Read the model definition and answer for the solid it produces. Units are mm, in the model's axes. Give positions to 0.01 mm unless a question says otherwise; leave off trailing zeros. Loops run counter-clockwise (first coordinate to the right, second up) from the corner with the lowest first, then second, coordinate; pieces in that order, holes last. Notation, with made-up numbers: (-25.5, -13) - (-15.5, -13) arc R18 ccw to (-15.5, 11) - close; hole circle Ø7 at (35, -37.75). An arc over 180 degrees is marked (long way). Put each result on its own line as item: value. Start each with the question number.
1. A cutting plane is placed at A-A, the plane y = 27. Determine the outline of the cut face in (x, z), plus the area to 3 significant figures.
2. Consider L1, parallel to Y at x = 0.45, z = -5.5; L2, parallel to Z at x = 0.5, y = 58.5; L3, parallel to Y at x = 0.95, z = -70.5. Determine where each line is inside the solid, lowest interval first. Write a range as from..to.
3. For a pull along Y with two mould halves and no side action, classify faces 1 (the flat face through (1.5, 15.6, -45.2)), 2 (the flat face through (0.76, 51.077, -11.662)) as released by +Y, released by -Y, zero draft, split by the parting line, or undercut.
4. A cutting plane is placed at C-C, the plane y = 63. Determine the outline of the cut face in (x, z), plus the area to 3 significant figures.
5. A cutting plane is placed at B-B, the plane x = 1.1. Count the separate pieces of the cut face and the enclosed holes in it, plus the area to 3 significant figures.
6. Given pin 1 Ø0.8 at (x, z) = (0.5, -44.5) entering from +Y, flat-ended and moving along its own axis, determine where the tip first touches the part or whether it passes through.
```python
from build123d import *

# Parameters (mm, degrees)
SKETCH1_R           = 1.05
BOSS_EXTRUDE1_DEPTH = 1.5
FILLET1_R           = 1.5
SKETCH2_W           = 117
SKETCH2_H           = 16
BOSS_EXTRUDE2_DEPTH = 1.5
CUT_EXTRUDE2_DEPTH  = 140.253366207
FILLET3_R           = 1
CUT_EXTRUDE3_DEPTH  = 140.253366207
BOSS_EXTRUDE3_DEPTH = 1.5
FILLET5_R           = 1.5


with BuildPart() as part:
    # Sketch1 → Boss-Extrude1 (new body)
    with BuildSketch(Plane(origin=(0, 0, 0), x_dir=(0, 0, -1), z_dir=(1, 0, 0))):
        Polygon((0, 0), (0, 75.5), (21.5, 75.5), (40, 0), (35.881667859, 0), (29.755840045, 25), (4, 25), (4, 0), align=None)
        with Locations((5.5, 72.5)):
            Circle(SKETCH1_R, mode=Mode.SUBTRACT)
        with Locations((18.5, 72.5)):
            Circle(SKETCH1_R, mode=Mode.SUBTRACT)
        Polygon((4, 69.5), (18.851866535, 69.5), (4, 29), align=None, mode=Mode.SUBTRACT)
        Polygon((8.260475549, 29), (20.558388216, 62.535546651), (28.775707595, 29), align=None, mode=Mode.SUBTRACT)
    extrude(amount=BOSS_EXTRUDE1_DEPTH)

    # Fillet1
    fillet1_edges = [part.edges().sort_by_distance(p)[0] for p in [
        (0.75, 75.5, -21.5),
        (0.75, 25, -29.755840045),
        (0.75, 25, -4),
        (0.75, 69.5, -4),
        (0.75, 29, -4),
        (0.75, 69.5, -18.851866535),
        (0.75, 29, -8.260475549),
        (0.75, 29, -28.775707595),
        (0.75, 62.535546651, -20.558388216),
    ]]
    fillet(fillet1_edges, radius=FILLET1_R)

    # Sketch2 → Boss-Extrude2 (add)
    with BuildSketch(Plane(origin=(1.5, 0, 0), x_dir=(0, 0, -1), z_dir=(1, 0, 0))):
        with Locations((58.5, 8)):
            Rectangle(SKETCH2_W, SKETCH2_H)
    extrude(amount=-BOSS_EXTRUDE2_DEPTH)

    # Sketch5 → Cut-Extrude2 (cut, through all)
    with BuildSketch(Plane(origin=(1.5, 0, 0), x_dir=(0, 0, -1), z_dir=(1, 0, 0))):
        Polygon((4.5, 11.5), (15.827584811, 11.5), (4.5, 5.626437506), align=None)
        Polygon((112.5, 11.5), (112.5, 5.626437506), (101.172415189, 11.5), align=None)
        Polygon((6.672415189, 4.5), (29.327584811, 4.5), (18, 10.373562494), align=None)
        Polygon((33.672415189, 4.5), (56.327584811, 4.5), (45, 10.373562494), align=None)
        Polygon((60.672415189, 4.5), (83.327584811, 4.5), (72, 10.373562494), align=None)
        Polygon((87.672415189, 4.5), (110.327584811, 4.5), (99, 10.373562494), align=None)
        Polygon((20.172415189, 11.5), (42.827584811, 11.5), (31.5, 5.626437506), align=None)
        Polygon((47.172415189, 11.5), (69.827584811, 11.5), (58.5, 5.626437506), align=None)
        Polygon((85.5, 5.626437506), (96.827584811, 11.5), (74.172415189, 11.5), align=None)
    extrude(amount=-CUT_EXTRUDE2_DEPTH, mode=Mode.SUBTRACT)

    # Fillet3
    fillet3_edges = [part.edges().sort_by_distance(p)[0] for p in [
        (0.75, 4.5, -56.327584811),
        (0.75, 4.5, -33.672415189),
        (0.75, 10.373562494, -45),
        (0.75, 5.626437506, -58.5),
        (0.75, 11.5, -47.172415189),
        (0.75, 11.5, -69.827584811),
        (0.75, 4.5, -29.327584811),
        (0.75, 4.5, -6.672415189),
        (0.75, 10.373562494, -18),
        (0.75, 5.626437506, -31.5),
        (0.75, 11.5, -20.172415189),
        (0.75, 11.5, -42.827584811),
        (0.75, 4.5, -110.327584811),
        (0.75, 4.5, -87.672415189),
        (0.75, 10.373562494, -99),
        (0.75, 5.626437506, -112.5),
        (0.75, 11.5, -101.172415189),
        (0.75, 11.5, -112.5),
        (0.75, 4.5, -83.327584811),
        (0.75, 4.5, -60.672415189),
        (0.75, 10.373562494, -72),
        (0.75, 5.626437506, -85.5),
        (0.75, 11.5, -74.172415189),
        (0.75, 11.5, -96.827584811),
        (0.75, 5.626437506, -4.5),
        (0.75, 11.5, -4.5),
        (0.75, 11.5, -15.827584811),
    ]]
    fillet(fillet3_edges, radius=FILLET3_R)

    # Sketch6 → Cut-Extrude3 (cut, through all)
    with BuildSketch(Plane(origin=(1.5, 0, 0), x_dir=(0, 0, -1), z_dir=(1, 0, 0))):
        Polygon((30.998526841, 19.928494428), (18.851866535, 69.5), (4, 69.5), (4, 19.75), align=None)
    extrude(amount=-CUT_EXTRUDE3_DEPTH, mode=Mode.SUBTRACT)

    # Sketch7 → Boss-Extrude3 (add)
    with BuildSketch(Plane(origin=(1.5, 0, 0), x_dir=(0, 0, -1), z_dir=(1, 0, 0))):
        Polygon((16.776232149, 69.5), (4, 23.476934928), (4, 16), (6.075634386, 16), (19.825004849, 65.528543637), (18.851866535, 69.5), align=None)
    extrude(amount=-BOSS_EXTRUDE3_DEPTH)

    # Fillet5
    fillet5_edges = [part.edges().sort_by_distance(p)[0] for p in [
        (0.75, 16, -31.961138058),
        (0.75, 16, -36.079470199),
        (0.75, 69.5, -4),
        (0.75, 69.5, -16.776232149),
        (0.75, 23.476934928, -4),
        (0.75, 16, -6.075634386),
        (0.75, 65.528543637, -19.825004849),
    ]]
    fillet(fillet5_edges, radius=FILLET5_R)


solid = part.part
```
Return value:
1. outline: (0, -33.38) - (1.5, -33.38) - (1.5, -29.27) - (0, -29.27) - close; (0, -9.13) - (1.5, -9.13) - (1.5, 0) - (0, 0) - close
1. area: 19.9 mm2
2. L1: y = 0..6.27, 11.5..32.99, 69.5..71.45, 73.55..75.5
2. L2: z = -25.67..-21.55, -17.87..-13.72, -4..0
2. L3: y = 0..4.5, 9.6..16
3. face 1: zero draft
3. face 2: undercut
4. outline: (0, -24.56) - (1.5, -24.56) - (1.5, -14.97) - (0, -14.97) - close; (0, -4) - (1.5, -4) - (1.5, 0) - (0, 0) - close
4. area: 20.4 mm2
5. separate pieces: 1
5. enclosed holes: 13
5. area: 2,180 mm2
6. pin 1: stops at y = 16
